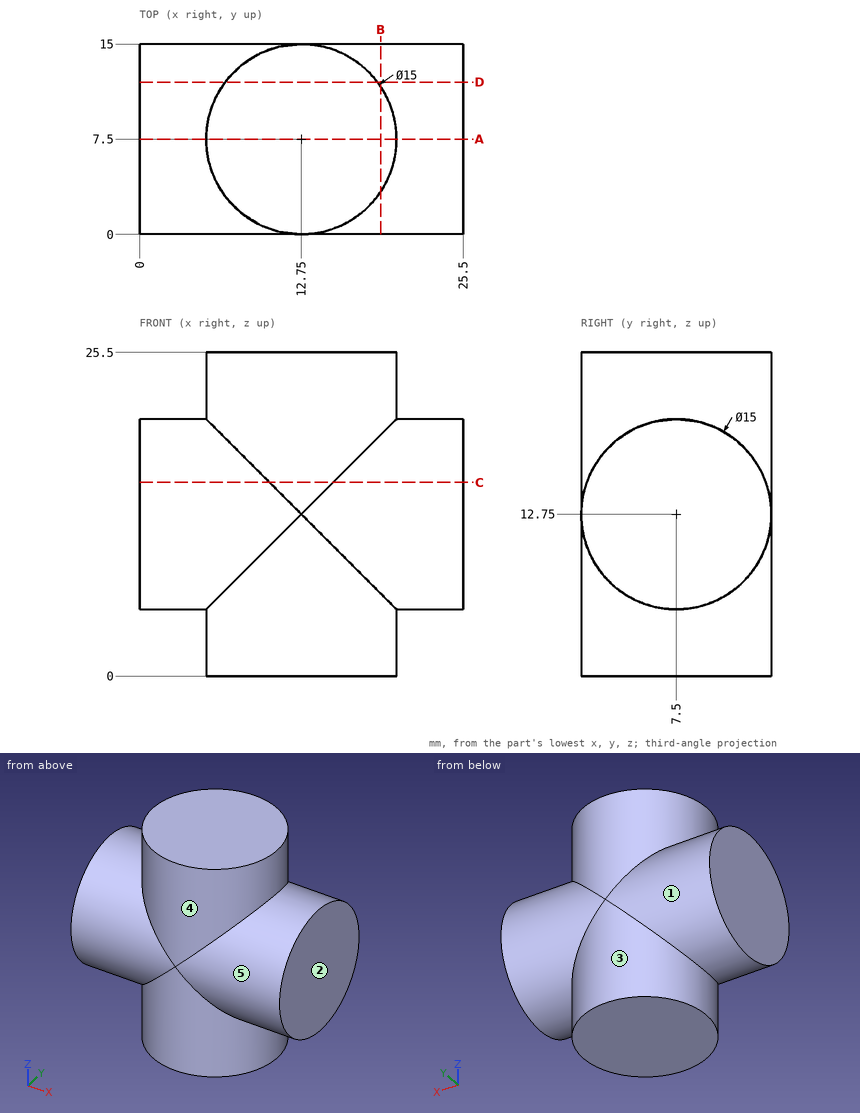
Could you check a few things on this drawing? It's one solid part, dimensions in mm from its lowest x, y, z. A direction names the side the tool comes from. Coordinates: 2 decimals unless noted, no trailing zeros. Write each loop counter-clockwise with the first axis right and the second up, starting at its lowest first coordinate (ties: lowest second). Pieces come first, ordered by that corner, then holes. Notation, with made-up numbers: (33, -22) - (71, -22) arc R21 cw to (71, 12) - close; hole circle Ø11 at (72, -7.75). An arc over 180 degrees is marked (long way). Write item = value, one per line.
1) Suppose I cut it at B-B on x = 19. Please give me the cut outline in (y, z).
Result set:
outline = (3.35, 0) - (11.65, 0) - (11.65, 6.5) arc R7.5 ccw to (11.65, 19) - (11.65, 25.5) - (3.35, 25.5) - (3.35, 19) arc R7.5 ccw to (3.35, 6.5) - close
2) Please list where these lines run through material, in increasing order: line 1 (Y direction, x = 12.5, z = 17.25); line 2 (Y direction, x = 5, z = 6.25); line 3 (X direction, y = 10, z = 20). Write a range as [from, to].
Result set:
line_1 = [0, 15]
line_2 = [3.76, 11.24]
line_3 = [5.68, 19.82]
3) Suppose I cut it at D-D on y = 12. Please give me the cut outline in (x, z), plus the area to 3 significant figures.
Result set:
outline = (0, 6.75) - (6.75, 6.75) - (6.75, 0) - (18.75, 0) - (18.75, 6.75) - (25.5, 6.75) - (25.5, 18.75) - (18.75, 18.75) - (18.75, 25.5) - (6.75, 25.5) - (6.75, 18.75) - (0, 18.75) - close
area = 468 mm2
4) Will these pins go through, and if not, where does the flat tip stop? pin 1 Ø1.5 at (x, z) = (9.5, 6) entering from +Y; pin 2 Ø2 at (x, z) = (16.5, 14.5) entering from +Y; pin 3 Ø1.5 at (x, z) = (15, 17.5) entering from +Y.
Result set:
pin_1 = 14.57
pin_2 = 14.96
pin_3 = 14.85
5) Suppose I cut it at C-C on z = 15.25. Please give me the cut outline in (x, y), plus the area to 4 significant figures.
Result set:
outline = (0, 0.43) - (10.25, 0.43) arc R7.5 ccw to (15.25, 0.43) - (25.5, 0.43) - (25.5, 14.57) - (15.25, 14.57) arc R7.5 ccw to (10.25, 14.57) - (0, 14.57) - close
area = 363.5 mm2
6) For the marked faces 1, 2, 3, 4 and 5, which set-ups out of +Z, -Z, +X, -X, +Y, -Y let a thin tool reach every point of the face, with its end or its side?
Result set:
face_1 = -X
face_2 = +Z, -Z, +X, +Y, -Y
face_3 = -Z
face_4 = +Z
face_5 = +X
7) Suppose I cut it at A-A on y = 7.5. Please give me the cut outline in (x, z).
Result set:
outline = (0, 5.25) - (5.25, 5.25) - (5.25, 0) - (20.25, 0) - (20.25, 5.25) - (25.5, 5.25) - (25.5, 20.25) - (20.25, 20.25) - (20.25, 25.5) - (5.25, 25.5) - (5.25, 20.25) - (0, 20.25) - close
